```python
from build123d import *
from build123d.topology import SkipClean

# Parameters (mm, degrees)
SKETCH1_R               = 25
BOSS_EXTRUDE1_DEPTH     = 5
SKETCH2_R               = 5
BOSS_EXTRUDE2_DEPTH     = 2
BOSS_EXTRUDE3_START     = 40
BOSS_EXTRUDE3_DEPTH     = 40
CUT_EXTRUDE1_DEPTH      = 69.255637517
CUT_EXTRUDE1_DEPTH_BACK = 69.255637517
SKETCH6_R               = 5


with BuildPart() as part:
    # Sketch1 → Boss-Extrude1 (new body)
    with BuildSketch(Plane.XY):
        Circle(SKETCH1_R)
    extrude(amount=BOSS_EXTRUDE1_DEPTH)

    # Sketch2 → Boss-Extrude2 (add)
    with BuildSketch(Plane.XY.offset(5)):
        with BuildLine():
            ThreePointArc((-1.427876097, -7.660444431), (-4.71777538, -2.961981327), (-10.258098312, -4.446506383))
            Line((-10.258098312, -4.446506383), (-2.597653881, -10.87438248))
            ThreePointArc((-2.597653881, -10.87438248), (-1.729412993, -9.370545148), (-1.427876097, -7.660444431))
        make_face()
        with BuildLine():
            Line((-2.597653881, -10.87438248), (-10.258098312, -4.446506383))
            ThreePointArc((-10.258098312, -4.446506383), (-9.641814145, -11.490666647), (-2.597653881, -10.87438248))
        make_face()
        with Locations((6.427876097, 7.660444431)):
            Circle(SKETCH2_R)
    extrude(amount=BOSS_EXTRUDE2_DEPTH)

    # Sketch3 → Boss-Extrude3 (add)
    with SkipClean():  # the faces are left unmerged after this step: merging them gives an invalid solid
        with BuildSketch(Plane(origin=(0, 0, 0), x_dir=(-1, 0, 0), z_dir=(0, 0, -1)).offset(BOSS_EXTRUDE3_START)):
            with BuildLine():
                Line((-24.346418841, 5.679074717), (-1.365085547, 24.962703008))
                ThreePointArc((-1.365085547, 24.962703008), (-16.069690242, 19.151111078), (-24.346418841, 5.679074717))
            make_face()
            with BuildLine():
                ThreePointArc((1.365085547, -24.962703008), (16.069690242, -19.151111078), (24.346418841, -5.679074717))
                Line((24.346418841, -5.679074717), (1.365085547, -24.962703008))
            make_face()
        extrude(amount=-BOSS_EXTRUDE3_DEPTH)

    # Sketch6 → Cut-Extrude1 (cut, two sides: drawn at the far end of the back side and taken through both)
    with SkipClean():  # the faces are left unmerged after this step: merging them gives an invalid solid
        with BuildSketch(Plane(origin=(12.855752194, 15.320888862, 0), x_dir=(0.7660444431189768, -0.642787609686541, 0), z_dir=(-0.642787609686541, -0.7660444431189768, 0)).offset(-CUT_EXTRUDE1_DEPTH_BACK)):
            with Locations((0, -28)):
                Circle(SKETCH6_R)
        extrude(amount=CUT_EXTRUDE1_DEPTH + CUT_EXTRUDE1_DEPTH_BACK, mode=Mode.SUBTRACT)


solid = part.part
```
Part model, mm, in its own coordinate system. A direction names the side the tool comes from. Round coordinates to 2 decimals unless told otherwise and drop trailing zeros. Loops run counter-clockwise (first coordinate to the right, second up) from the corner with the lowest first, then second, coordinate; pieces in that order, holes last.
Item 1: Cut at D-D, the plane z = 1.5. Give the cut face in (x, y), then the cut area to 3 significant figures.
Item 2: 3-axis set-ups, long thin cutter, end or side, ignore diameter. For faces 1 (the face through (14, 16, -40)), 2 (the face through (13, 15.2, -20.3)), 3 (the face through (-13, -15.2, -20.3)), 4 (the face through (0, 0, 5)): which of +Z, -Z, +X, -X, +Y, -Y reach the whole face in a straight line?
Item 3: Cut at A-A, the plane z = -36.5. Give the cut face in (x, y).
Item 4: Mould opens along Z. For faces 5 (the face through (0, 0, 0)), 6 (the face through (-6, -8, 7)), 7 (the face through (18.02, 14.29, -29.92)) say: +Z half, -Z half, draft (parallel to the pull), parting line (faces both ways), or undercut.
Item 5: Drill centre lines: line 1 (Z direction, x = -14.5, y = 3.5); line 2 (Z direction, x = 13, y = 20.5); line 3 (Y direction, x = 10, z = -3). Where is each one in solid material? Low to high.
Item 6: Cut at B-B, the plane x = -6. Give the cut face in (y, z), then the cut area to 3 significant figures.
Item 7: Drop flat-ended pins along their axis: P1, Ø6, axis at y = -1, z = -1, coming from the -X side; P2, Ø2, axis at x = -4, y = 13.5, coming from the +Z side; P3, Ø6, axis at x = 5, z = -16.5, coming from the +Y side; P4, Ø1.5, axis at x = -6.5, z = -1.5, coming from the -Y side. Give the stop position or say it passes through.
Item 8: Cut at C-C, the plane y = -3.5. Give the cut face in (x, z), then the cut area to 3 significant figures.
A:
1. outline: circle Ø50 at (0, 0)
1. area: 1,960 mm2
2. face 1: -Z, +X, -X, +Y, -Y
2. face 2: -Z, -X, -Y
2. face 3: -Z, +X, +Y
2. face 4: +Z
3. outline: (-24.35, -5.68) arc R25 ccw to (-1.37, -24.96) - close; (1.37, 24.96) - (24.35, 5.68) arc R25 ccw to start
4. face 5: -Z half
4. face 6: +Z half
4. face 7: undercut
5. line 1: z = 0 to 5
5. line 2: z = -40 to -31.83, -24.17 to 5
5. line 3: y = 17.72 to 22.91
6. outline: (-24.27, -40) - (-21.07, -40) - (-21.07, 0) - (24.27, 0) - (24.27, 5) - (-2.68, 5) - (-2.68, 7) - (-12.64, 7) - (-12.64, 5) - (-24.27, 5) - close
6. area: 390 mm2
7. P1: stops at x = -25
7. P2: stops at z = 5
7. P3: stops at y = 24.92
7. P4: stops at y = -24.33
8. outline: (-24.75, 0) - (24.75, 0) - (24.75, 5) - (-3.65, 5) - (-3.65, 7) - (-9.2, 7) - (-9.2, 5) - (-24.75, 5) - close
8. area: 259 mm2
